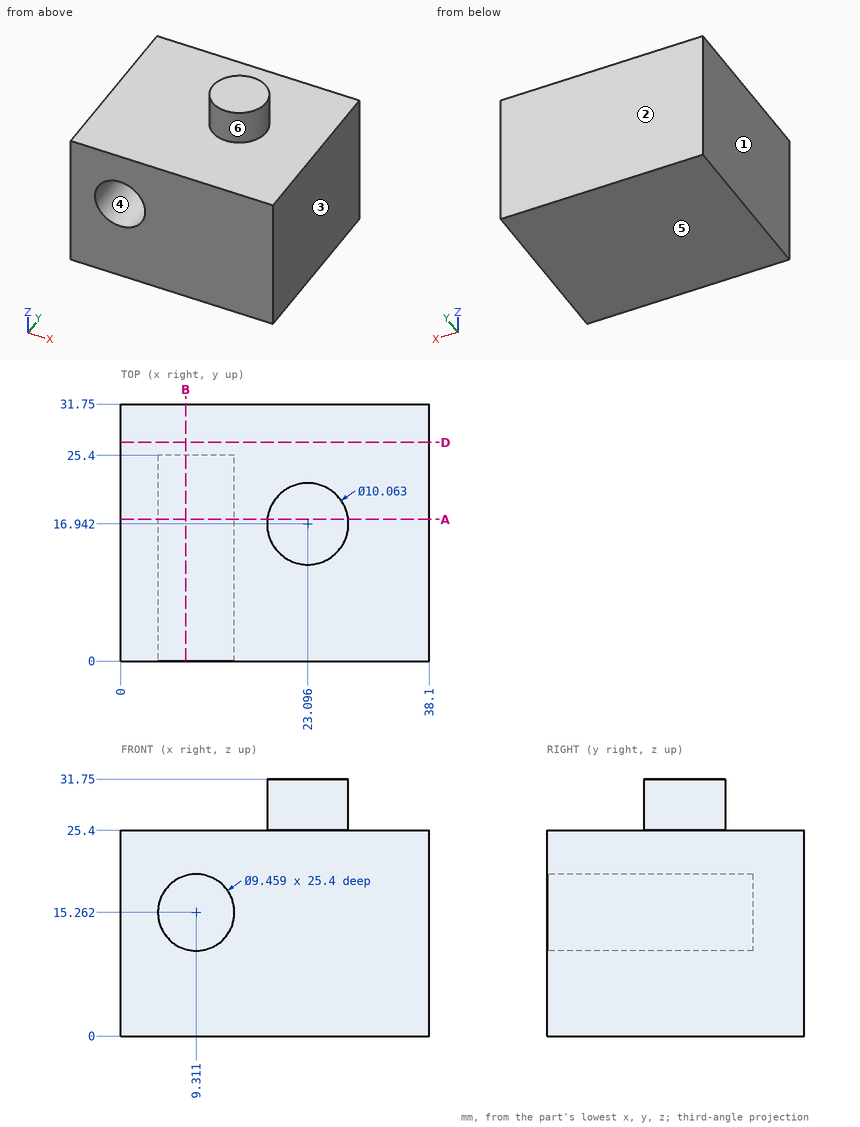
Here's the drawing with two shaded views (mm, measured from the low corner). I have some questions. A direction names the side the tool comes from. Round coordinates to 2 decimals unless told otherwise and drop trailing zeros. Loops run counter-clockwise (first coordinate to the right, second up) from the corner with the lowest first, then second, coordinate; pieces in that order, holes last. Notation, with made-up numbers: M -23.75,-25 L 16.25,-25 A32 cw 16.25,10 Z; hole C 18.5,-3.5 d6. An arc over 180 degrees is marked long. Put each result on its own line as item: value.
Q1. Imagine slicing it at A-A (y = 17.5). Write out the boundary of the cut face in (x, z), then the cut area to 3 significant figures.
Check result:
outline: M 0,0 L 38.1,0 L 38.1,25.4 L 28.1,25.4 L 28.1,31.75 L 18.1,31.75 L 18.1,25.4 L 0,25.4 Z; hole C 9.31,15.26 d9.46
area: 961 mm2
Q2. For pin 1 (1.5 mm diameter, centred on x = 7.5, z = 12.5, fed in from -Y); pin 2 (8 mm diameter, centred on x = 9, y = 11, fed in from +Z), each with a flat end and sliding along its axis, tell me the tip position at first contact or that it passes through.
Check result:
pin 1: y = 25.4
pin 2: z = 25.4
Q3. Imagine slicing it at B-B (x = 8). Write out the boundary of the cut face in (y, z).
Check result:
outline: M 0,0 L 31.75,0 L 31.75,25.4 L 0,25.4 L 0,19.81 L 25.4,19.81 L 25.4,10.72 L 0,10.72 Z
Q4. I need wall thicknesses on probe 1 along Z at (x, y) = (7, 4) (1 decimal); probe 2 along Z at (x, y) = (32, 20.5); probe 3 along Z at (x, y) = (7.5, 14.5). Which ranges of each line are inside material? Lowest first, please.
Check result:
probe 1: 0 to 11.1, 19.4 to 25.4
probe 2: 0 to 25.4
probe 3: 0 to 10.89, 19.63 to 25.4
Q5. Imagine slicing it at D-D (y = 27). Write out the boundary of the cut face in (x, z), then the cut area to 3 significant figures.
Check result:
outline: M 0,0 L 38.1,0 L 38.1,25.4 L 0,25.4 Z
area: 968 mm2
Q6. On a 3-axis mill with a long thin cutter (end or side, diameter ignored), from which of +Z, -Z, +X, -X, +Y, -Y can I reach the whole of each face in a straight line? I mean the marked faces 5 and 6. Say none if no direction works.
Check result:
face 5: -Z, +X, -X, +Y, -Y
face 6: +Z
Q7. Thinking about a two-plate mould opening in X: for the marked faces 1, 2, 3 and 4, which applies, released by +X, released by -X, zero draft, split by the parting line, or undercut?
Check result:
face 1: released by -X
face 2: zero draft
face 3: released by +X
face 4: undercut
